Design review of the part built by this model. Coordinates are the model's own, in mm. Coordinates: 2 decimals unless noted, no trailing zeros. Order: outer loops, then holes, each group sorted by start corner. A loop starts at its lowest first (then second) coordinate and runs counter-clockwise, first axis right, second up. Notation, with made-up numbers: (-17.75, -29) -> (20.25, -29) arc R21 cw to (20.25, -12) -> close; hole circle Ø3 at (56.5, 46.25). An arc over 180 degrees is marked (long way). Write item = value, one per line.
```python
from build123d import *

# Parameters (mm, degrees)
BOSS_EXTRUDE1_DEPTH = 5


with BuildPart() as part:
    # Sketch2 → Boss-Extrude1 (new body)
    with BuildSketch(Plane.XY.offset(324.609115736)):
        with BuildLine():
            Line((-16.90012844, -8.183190187), (72.816503584, -45.112441184))
            Line((72.816503584, -45.112441184), (74.339048342, -41.413541691))
            Line((74.339048342, -41.413541691), (78.962672709, -43.316722639))
            Line((78.962672709, -43.316722639), (81.627126035, -36.843648526))
            Line((81.627126035, -36.843648526), (77.003501669, -34.940467578))
            Line((77.003501669, -34.940467578), (79.287318806, -29.392118339))
            Line((79.287318806, -29.392118339), (83.910943172, -31.295299286))
            Line((83.910943172, -31.295299286), (86.575396499, -24.822225173))
            Line((86.575396499, -24.822225173), (81.951772132, -22.919044226))
            Line((81.951772132, -22.919044226), (83.47431689, -19.220144733))
            Line((83.47431689, -19.220144733), (-6.242315134, 17.709106264))
            add(Edge.make_bspline(
                [(-6.242315134, 17.709106264), (-19.147085678, 28.427579084), (-62.609683594, 83.624540664), (-113.341454038, 133.123455083), (-159.667254415, 160.823469136)],
                knots=[0, 0, 0, 0, 0.237148473, 1, 1, 1, 1], degree=3))
            add(Edge.make_bspline(
                [(-192.022205471, 204.724702407), (-183.525718419, 177.076811357), (-159.667254415, 160.823469136)],
                knots=[0, 0, 0, 1, 1, 1], degree=2))
            Line((-192.022205471, 204.724702407), (-204.287606756, 174.926900827))
            Line((-204.287606756, 174.926900827), (-208.911231122, 176.830081774))
            Line((-208.911231122, 176.830081774), (-219.569044429, 150.937785322))
            Line((-219.569044429, 150.937785322), (-214.945420062, 149.034604375))
            Line((-214.945420062, 149.034604375), (-224.18290752, 126.592874832))
            add(Edge.make_bspline(
                [(-175.911850273, 128.697068335), (-200.797987469, 136.066038881), (-224.18290752, 126.592874832)],
                knots=[0, 0, 0, 1, 1, 1], degree=2))
            add(Edge.make_bspline(
                [(-16.90012844, -8.183190187), (-30.222192507, 2.01197393), (-75.852029724, 55.431258283), (-128.517955825, 102.867060046), (-175.911850273, 128.697068335)],
                knots=[0, 0, 0, 0, 0.237148473, 1, 1, 1, 1], degree=3))
        make_face()
        with BuildLine():
            Line((65.049758472, -17.908345143), (-8.450005033, 12.345702))
            add(Edge.make_bspline(
                [(-8.450005033, 12.345702), (-21.566591824, 22.803900379), (-66.124581019, 77.120450197), (-117.836312175, 125.594689972), (-164.70691842, 152.362521961)],
                knots=[0, 0, 0, 0, 0.237148473, 1, 1, 1, 1], degree=3))
            ThreePointArc((-164.70691842, 152.362521961), (-175.410879134, 147.900994755), (-170.949351927, 137.19703404))
            add(Edge.make_bspline(
                [(-14.692438541, -2.819785922), (-27.809025332, 7.638412457), (-72.367014526, 61.954962275), (-124.078745683, 110.429202051), (-170.949351927, 137.19703404)],
                knots=[0, 0, 0, 0, 0.237148473, 1, 1, 1, 1], degree=3))
            Line((-14.692438541, -2.819785922), (58.807324964, -33.073833065))
            Line((58.807324964, -33.073833065), (65.049758472, -17.908345143))
        make_face(mode=Mode.SUBTRACT)
    extrude(amount=-BOSS_EXTRUDE1_DEPTH)


solid = part.part
```
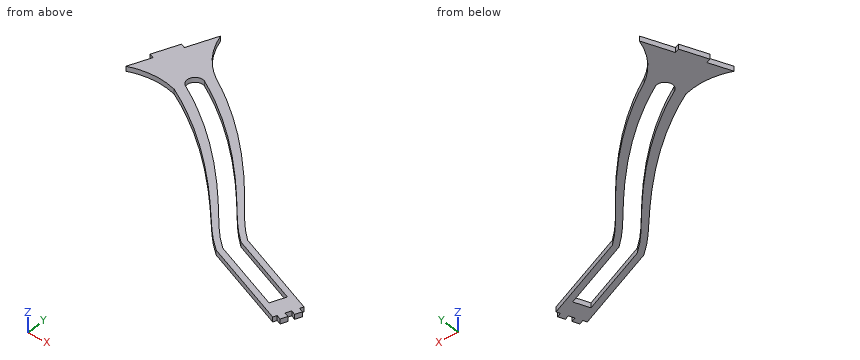
(1) Insertion check: pin 1 (3 mm diameter, centred on y = 1, z = 323.5, fed in from +X); pin 2 (3 mm diameter, centred on x = -188, z = 324, fed in from +Y); pin 3 (1.5 mm diameter, centred on y = 163.5, z = 321, fed in from +X). Each pin has a flat end and moves straight along its axis. Give the tip position at first contact, or say it passes through.
Report:
pin_1 = 38
pin_2 = 197.6
pin_3 = -162.39
(2) For L1, parallel to Y at x = 31, z = 320; L2, parallel to Y at x = -126.5, z = 323.4; L3, parallel to X at y = 36.5, z = 321.9, list the stretches that pass through material, from the lowest coordinate up.
Report:
L1 = -27.9 to -21.63, -3.89 to 2.38
L2 = 96.42 to 107.33, 127.25 to 138.42
L3 = -61.04 to -52.36, -32.88 to -25.15
(3) We need section A-A (x = 21.5). Write out the cut boundary in (y, z).
Report:
outline = (-23.99, 319.61) -> (-17.72, 319.61) -> (-17.72, 324.61) -> (-23.99, 324.61) -> close; (0.02, 319.61) -> (6.29, 319.61) -> (6.29, 324.61) -> (0.02, 324.61) -> close
